Geometry: final body of the model. Coordinates: model frame, mm. A direction names the side the tool comes from. Round coordinates to 2 decimals unless told otherwise and drop trailing zeros. Write each loop counter-clockwise with the first axis right and the second up, starting at its lowest first coordinate (ties: lowest second). Pieces come first, ordered by that corner, then holes. Notation, with made-up numbers: M -23,33 L 20,33 A30 cw 20,62 Z; hole C 81.25,56.5 d4. An arc over 180 degrees is marked long. Put each result on its own line as item: value. Start each with the question number.
```python
from build123d import *

# Parameters (mm, degrees)
BOSS_EXTRUDE1_DEPTH     = 24
SKETCH2_R               = 12
SKETCH2_R_2             = 7
BOSS_EXTRUDE2_DEPTH     = 20
CUT_EXTRUDE1_DEPTH      = 70.397406292
CUT_EXTRUDE1_DEPTH_BACK = 70.397406292
SKETCH3_R               = 7


with BuildPart() as part:
    # Sketch1 → Boss-Extrude1 (new, symmetric)
    with BuildSketch(Plane.XY):
        Polygon((0, 0), (44, 0), (44, 47.073103448), (44, 48), (36, 48), (36, 8), (8, 8), (8, 48), (0, 48), align=None)
    extrude(amount=BOSS_EXTRUDE1_DEPTH, both=True)

    # Sketch2 → Boss-Extrude2 (add)
    with BuildSketch(Plane(origin=(44, 0, 0), x_dir=(0, 0, -1), z_dir=(1, 0, 0))):
        with Locations(Location((0, 24, 0), (0, 0, 180))):
            Circle(SKETCH2_R)
        with Locations((0, 24)):
            Circle(SKETCH2_R_2, mode=Mode.SUBTRACT)
    boss_extrude2 = extrude(amount=BOSS_EXTRUDE2_DEPTH)

    # Sketch3 → Cut-Extrude1 (cut, two sides: drawn at the far end of the back side and taken through both)
    with BuildSketch(Plane(origin=(44, 0, 0), x_dir=(0, 0, -1), z_dir=(1, 0, 0)).offset(-CUT_EXTRUDE1_DEPTH_BACK)):
        with Locations((0, 24)):
            Circle(SKETCH3_R)
    extrude(amount=CUT_EXTRUDE1_DEPTH + CUT_EXTRUDE1_DEPTH_BACK, mode=Mode.SUBTRACT)

    # Mirror1: Boss-Extrude2 across plane
    add(boss_extrude2.mirror(Plane.ZY.offset(-22)))


solid = part.part
```
1) Section B-B, the plane z = 0. Output: boundary loops of the cut face in (x, y), and give its area (3 significant figures).
2) Section D-D, the plane x = 2. Output: boundary loops of the cut face in (y, z).
3) Draft query along Y for faces 1 (the face through (8, 32, 0)), 2 (the face through (49.804, 17.166, 1.517)), 3 (the face through (-9.86, 12.1, -1.56)). Return one class per face: +Y half, -Y half, draft (parallel to the pull), parting line (faces both ways), or undercut.
4) Section A-A, the plane y = 24. Output: boundary loops of the cut face in (x, z).
5) Ray query, probe 1 along X at (y, z) = (29.5, 15.5); probe 2 along Z at (x, y) = (2.75, 24); probe 3 along Z at (x, y) = (-7.25, 24). Return the intervals inside material, ascending.
6) Section C-C, the plane y = 41. Output: boundary loops of the cut face in (x, z).
7) First-contact query: pin 1 (4 mm diameter, centred on y = 21, z = 3.5, fed in from +X); pin 2 (3 mm diameter, centred on x = 54.5, y = 19, fed in from -Z); pin 3 (5 mm diameter, centred on y = 8.5, z = -19, fed in from +X). Flat tips, straight axial feed; report the tip coordinate or a pass-through.
8) Access query for faces 4 (the face through (36, 33, 0)), 5 (the face through (7, 24, 24)), 6 (the face through (0, 35, 6)), 7 (the face through (53.86, 12.1, -1.56)). Directions: +Z, -Z, +X, -X, +Y, -Y. A direction counts if a zero-diameter tool reaches every point of the face in a straight line with its end or side. Return the directions, or none.
Solved:
1. outline: M -20,12 L 0,12 L 0,0 L 44,0 L 44,12 L 64,12 L 64,17 L 36,17 L 36,8 L 8,8 L 8,17 L -20,17 Z; M -20,31 L 8,31 L 8,48 L 0,48 L 0,36 L -20,36 Z; M 36,31 L 64,31 L 64,36 L 44,36 L 44,48 L 36,48 Z
1. area: 1,170 mm2
2. outline: M 0,-24 L 48,-24 L 48,24 L 0,24 Z; hole C 24,0 d14
3. face 1: draft
3. face 2: undercut
3. face 3: parting line
4. outline: M -20,-12 L 0,-12 L 0,-24 L 8,-24 L 8,-7 L -20,-7 Z; M -20,7 L 8,7 L 8,24 L 0,24 L 0,12 L -20,12 Z; M 36,-24 L 44,-24 L 44,-12 L 64,-12 L 64,-7 L 36,-7 Z; M 36,7 L 64,7 L 64,12 L 44,12 L 44,24 L 36,24 Z
5. probe 1: x = 0 to 8, 36 to 44
5. probe 2: z = -24 to -7, 7 to 24
5. probe 3: z = -12 to -7, 7 to 12
6. outline: M 0,-24 L 8,-24 L 8,24 L 0,24 Z; M 36,-24 L 44,-24 L 44,24 L 36,24 Z
7. pin 1: passes through
7. pin 2: stops at z = -11.48
7. pin 3: stops at x = 44
8. face 4: +Z, -Z, +Y
8. face 5: +Z, +X, -X, +Y, -Y
8. face 6: -X
8. face 7: +X
